Autodesk Inventor part; units mm, degrees
ref_plane "YZ Plane" through (0, 0, 0) normal (1, 0, 0) x (0, 1, 0)
ref_plane "XZ Plane" through (0, 0, 0) normal (0, 1, 0) x (-1, 0, 0)
ref_plane "XY Plane" through (0, 0, 0) normal (0, 0, 1) x (1, 0, 0)
sketch "Sketch1" plane through (0, 0, 0) normal (0, 1, 0) x (-1, 0, 0)
  line L0 (20.25, -10) -> (-20.25, -10)
  line L1 (-20.25, -10) -> (-20.25, 10)
  line L2 (-20.25, 10) -> (20.25, 10)
  line L3 (20.25, 10) -> (20.25, -10)
  point P0 (0, 0)
  dimension "d0" = 40.5
  dimension "d1" = 20
  dimension "d2" = 10
  dimension "d3" = 20.25
extrude "Plate1" add sketch "Sketch1" along normal blind 1.5
sketch "Sketch2" plane through (21.75, 0, -10) normal (-1, 0, 0) x (0, -1, 0)
  line L0 (0, 20) -> (0, 0)
  line L1 (0, 0) -> (-50, 0)
  line L2 (-50, 0) -> (-50, 20)
  line L3 (-50, 20) -> (0, 20)
edge flange "Flange1" height 50 angle 90 thickness 1.5 bend radius 0.31 thickness toward (-1, 0, 0) relief tear relief width 1.5 relief depth 0.75 edges at (20.25, 1.5, 0) wall of the first edge with corners at (21.75, 0, 10) (21.75, 0, -10) (21.75, 50, -10) (21.75, 50, 10)
bend "Bend1"
corner "Corner1"
sketch "Sketch3" plane through (-21.75, 0, 10) normal (1, 0, 0) x (0, 1, 0)
  line L0 (0, -20) -> (0, 0)
  line L1 (0, 0) -> (50, 0)
  line L2 (50, 0) -> (50, -20)
  line L3 (50, -20) -> (0, -20)
edge flange "Flange2" height 50 angle 90 thickness 1.5 bend radius 0.31 thickness toward (1, 0, 0) relief tear relief width 1.5 relief depth 0.75 edges at (-20.25, 1.5, 0) wall of the first edge with corners at (-21.75, 0, -10) (-21.75, 0, 10) (-21.75, 50, 10) (-21.75, 50, -10)
bend "Bend2"
corner "Corner2"
sketch "Sketch4" plane through (21.75, 50, 10) normal (1, 0, 0) x (0, 0, -1)
  circle A0 centre (10, -9.9) radius 6.4
  line L0 (0, 0) -> (20, 0)
  line L1 (20, 0) -> (20, -48.19)
  point P0 (10, -50)
  dimension "d25" = 9.9
  dimension "d26" = 12.8
  dimension "d27" = 10
extrude "Extrusion1" cut sketch "Sketch4" against normal blind 50
sketch "Sketch5" plane through (21.75, 50, 10) normal (1, 0, 0) x (0, 0, -1)
  circle A0 centre (10, -9.9) radius 6.4
  line L0 (0, 0) -> (20, 0)
  line L1 (-4, 0) -> (24, 0)
  line L2 (24, 0) -> (24, -9.9)
  line L3 (24, -9.9) -> (-4, -9.9)
  line L4 (-4, -9.9) -> (-4, 0)
  line L5 (0, -48.19) -> (0, 0)
  point P0 (10, -50)
  dimension "d30" = 9.9
  dimension "d31" = 28
  dimension "d32" = 4
extrude "Extrusion2" cut sketch "Sketch5" against normal blind 50 contours L3 A0 | A0 L3 L5 L0 L1 L2 | L3 L4 L1 L5 picked at (9.2435, -7.9053)
fillet "Fillet1" radius 1 4 edges at (-21, 40.1, 10) (-21, 40.1, -10) (21, 40.1, -10) (21, 40.1, 10)
sketch "Sketch6" plane through (-21.75, 1.81, -10) normal (-1, 0, 0) x (0, 0, 1)
  circle A0 centre (18, 31.39) radius 0.7835
  circle A1 centre (2, 31.39) radius 0.7835
  circle A2 centre (3, 18.17) radius 0.7835
  circle A3 centre (17, 18.17) radius 0.7835
  circle A4 centre (10, 10.87) radius 0.7835
  point P0 (10, -1.81)
hole "Hole1" at (-21.75, 33.2, -8) at (-21.75, 19.98, -7) at (-21.75, 12.68, 0) at (-21.75, 33.2, 8) at (-21.75, 19.98, 7) direction (1, 0, 0) diameter 2.1 depth 1.5
sketch "Sketch7" plane through (21.75, 1.81, 10) normal (1, 0, 0) x (0, 0, -1)
  circle A0 centre (17.525, 25.79) radius 0.7835
  circle A1 centre (2.475, 25.79) radius 0.7835
  circle A2 centre (17.525, 10.69) radius 0.7835
  circle A3 centre (2.475, 10.69) radius 0.7835
  point P0 (10, -1.81)
hole "Hole2" at (21.75, 27.6, 7.525) at (21.75, 27.6, -7.525) at (21.75, 12.5, -7.525) at (21.75, 12.5, 7.525) direction (-1, 0, 0) diameter 2.1 depth 1.5
sketch "Sketch8" plane through (0, 0, 0) normal (0, -1, 0) x (1, 0, 0)
  circle A0 centre (8, -8) radius 1.05
  circle A1 centre (-8, -8) radius 1.05
  circle A2 centre (8, 8) radius 1.05
  circle A3 centre (-8, 8) radius 1.05
  point P0 (0, 0)
hole "Hole3" at (8, 0, -8) at (-8, 0, -8) at (-8, 0, 8) at (8, 0, 8) direction (0, 1, 0) diameter 2.1 depth 1.5
equation "\"d41\" = Thickness"
equation "\"d48\" = Thickness"
equation "\"d55\" = Thickness"
equation "\"d4\" = Thickness"
equation "\"d5\" = BendReliefWidth"
equation "\"d6\" = BendReliefDepth"
equation "\"d7\" = MinimumRemnant"
equation "\"d8\" = TransitionRadius"
equation "\"d11\" = BendRadius"
equation "\"d12\" = CornerReliefSize"
equation "\"d13\" = GapSize"
equation "\"d14\" = JacobiRadiusSize"
equation "\"d15\" = BendReliefWidth"
equation "\"d16\" = BendReliefDepth"
equation "\"d17\" = MinimumRemnant"
equation "\"d18\" = TransitionRadius"
equation "\"d21\" = BendRadius"
equation "\"d22\" = CornerReliefSize"
equation "\"d23\" = GapSize"
equation "\"d24\" = JacobiRadiusSize"
equation "\"BendReliefWidth\" = Thickness"
equation "\"BendReliefDepth\" = 0.5 * Thickness"
equation "\"CornerReliefSize\" = 4 * Thickness"
equation "\"MinimumRemnant\" = 2 * Thickness"
equation "\"TransitionRadius\" = BendRadius"
equation "\"JacobiRadiusSize\" = BendRadius"
equation "\"GapSize\" = Thickness"
properties part number "axis_10_top_frame" material "Aluminum 6061-AHC"
Geometry: final body of the model. Coordinates: model frame, mm. A direction names the side the tool comes from. Give positions to 0.01 mm unless a question says otherwise; leave off trailing zeros. Loops run counter-clockwise (first coordinate to the right, second up) from the corner with the lowest first, then second, coordinate; pieces in that order, holes last. Notation, with made-up numbers: (-6, -36) - (49, -36) arc R7 ccw to (49, -23) - close; hole circle Ø7 at (-13, -38.5). An arc over 180 degrees is marked (long way). One line per question, with ' | ' between items. Start each with the question number.
(1) Section query D-D on y = 23. Return loops of the section in (x, z), then the cut area to 3 significant figures.
(2) Contact query for flat-ended pins moving along their axis: pin 1 (1.9 mm diameter, centred on x = 8, z = 8, fed in from -Y); pin 2 (1.7 mm diameter, centred on y = 27.6, z = -7.525, fed in from +X); pin 3 (1.7 mm diameter, centred on y = 19.98, z = -7, fed in from -X). Output: stop coordinate, or through.
(3) Pull-direction query (Z, two-part tool) for faces 1 (the cylindrical face through (20.99, 11.615, -8.089)), 2 (the flat face through (0, 1.5, 0)), 3 (the cylindrical face through (-20.99, 32.16, -8.14)), 4 (the cylindrical face through (20.99, 39.799, 9.715)); classes: released by +Z, released by -Z, zero draft, split by the parting line, or undercut.
(4) Reachability of faces 5 (the cylindrical face through (20.99, 26.56, 7.66)), 6 (the flat face through (-20.25, 21, 0)), 7 (the flat face through (-21, 40.1, 8)) from +Z, -Z, +X, -X, +Y, -Y: full face, straight path, thin tool, end or side. Return the list, or none.
(5) Section query C-C on y = 27.6. Return loops of the section in (x, z) (3 decimals).
(6) Section query A-A on x = -8. Return loops of the section in (y, z), then the cut area to 3 significant figures.
(7) Ray query, line 1 (Z direction, x = -20.55, y = 19.98); line 2 (X direction, y = 18, z = 5.5); line 3 (Z direction, x = 20.8, y = 12.5) (3 decimals). Return the intervals inside material, ascending. Write a range as from..to.
(8) Section query B-B on z = 0. Return loops of the section in (x, y).
The answers:
1) outline: (-21.75, -10) - (-20.25, -10) - (-20.25, 10) - (-21.75, 10) - close; (20.25, -10) - (21.75, -10) - (21.75, 10) - (20.25, 10) - close | area: 60.0 mm2
2) pin 1: through | pin 2: x = -20.25 | pin 3: x = 20.25
3) face 1: undercut | face 2: zero draft | face 3: undercut | face 4: released by +Z
4) face 5: +X | face 6: +Z, -Z, +Y | face 7: +Z, -Z, +X, -X, +Y
5) outline: (-21.75, -10) - (-20.25, -10) - (-20.25, 10) - (-21.75, 10) - close; (20.25, -10) - (21.75, -10) - (21.75, -8.575) - (20.25, -8.575) - close; (20.25, -6.475) - (21.75, -6.475) - (21.75, 6.475) - (20.25, 6.475) - close; (20.25, 8.575) - (21.75, 8.575) - (21.75, 10) - (20.25, 10) - close
6) outline: (0, -10) - (1.5, -10) - (1.5, -9.05) - (0, -9.05) - close; (0, -6.95) - (1.5, -6.95) - (1.5, 6.95) - (0, 6.95) - close; (0, 9.05) - (1.5, 9.05) - (1.5, 10) - (0, 10) - close | area: 23.7 mm2
7) line 1: -10..-8.05, -5.95..5.95, 8.05..10 | line 2: -21.75..-20.25, 20.25..21.75 | line 3: -10..-8.575, -6.475..6.475, 8.575..10
8) outline: (-21.75, 1.81) arc R1.81 ccw to (-19.94, 0) - (19.94, 0) arc R1.81 ccw to (21.75, 1.81) - (21.75, 33.7) - (20.25, 33.7) - (20.25, 1.81) arc R0.31 cw to (19.94, 1.5) - (-19.94, 1.5) arc R0.31 cw to (-20.25, 1.81) - (-20.25, 11.63) - (-21.75, 11.63) - close; (-21.75, 13.73) - (-20.25, 13.73) - (-20.25, 33.7) - (-21.75, 33.7) - close
